Print and shaded views of the part. All mm, measured from the part's lowest x, y and z. A direction names the side the tool comes from. Coordinates: 2 decimals unless noted, no trailing zeros. Loops run counter-clockwise (first coordinate to the right, second up) from the corner with the lowest first, then second, coordinate; pieces in that order, holes last.
1) Wall check: line 1 along Y through (x, z) = (17.5, 1.75); line 2 along X through (y, z) = (7.5, 1.4); line 3 along X through (y, z) = (14.25, 1.45). Give the ranges that are in metal, low to high.
2) Saw through at C-C, the plane z = 1.4. Write the cut outline in (x, y), and give its area (3 significant figures).
3) Pin check, flat tips, straight feed: pin 1 Ø4 at (x, y) = (21, 3.5) entering from -Z; pin 2 Ø1.5 at (x, y) = (6, 6) entering from +Z (3 decimals). Stop position of each tip, or through.
4) Saw through at B-B, the plane y = 9.5. Write the cut outline in (x, z), and give its area (3 significant figures).
5) Saw through at A-A, the plane x = 20.75. Write the cut outline in (y, z).
6) Which spindle directions (+Z, -Z, +X, -X, +Y, -Y) get a long thin tool onto all of the face, cutting with end or side? Do the marked faces 1 and 2. Say none if no direction does.
7) Two-plate mould, pull along X, no slides. Class the marked faces 3, 4 and 5: +X half, -X half, draft (parallel to the pull), parting line (faces both ways), or undercut.
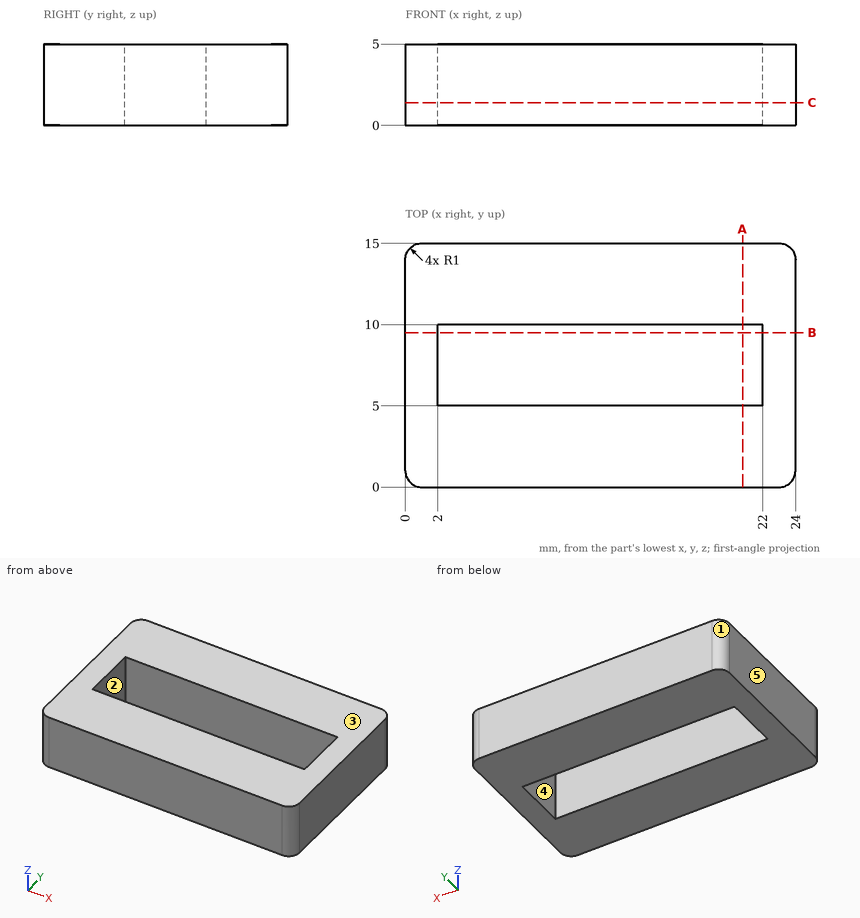
Data:
1. line 1: y = 0 to 5, 10 to 15
1. line 2: x = 0 to 2, 22 to 24
1. line 3: x = 0.03 to 23.97
2. outline: (0, 1) arc R1 ccw to (1, 0) - (23, 0) arc R1 ccw to (24, 1) - (24, 14) arc R1 ccw to (23, 15) - (1, 15) arc R1 ccw to (0, 14) - close; hole (2, 5) - (22, 5) - (22, 10) - (2, 10) - close
2. area: 259 mm2
3. pin 1: stops at z = 0
3. pin 2: passes through
4. outline: (0, 0) - (2, 0) - (2, 5) - (0, 5) - close; (22, 0) - (24, 0) - (24, 5) - (22, 5) - close
4. area: 20.0 mm2
5. outline: (0, 0) - (5, 0) - (5, 5) - (0, 5) - close; (10, 0) - (15, 0) - (15, 5) - (10, 5) - close
6. face 1: +Z, -Z, -X, +Y
6. face 2: +Z, -Z
7. face 3: draft
7. face 4: undercut
7. face 5: -X half
